Design review of the part shown in the three views and the two pictorial views. Dimensions are in mm from the part's minimum x, y and z. A direction names the side the tool comes from. Round coordinates to 2 decimals unless told otherwise and drop trailing zeros. Loops run counter-clockwise (first coordinate to the right, second up) from the corner with the lowest first, then second, coordinate; pieces in that order, holes last.
1. Tool access review of the marked faces 1 and 2: name each direction out of +Z, -Z, +X, -X, +Y, -Y from which nothing blocks a thin tool from reaching the whole face with its end or side.
2. Consider section D-D on z = 49. State the section outline as (x, y) points, then the cut area to 3 significant figures.
3. Clearance check with flat-ended pins moving along their axes: pin 1 Ø12 at (x, y) = (61, 33) entering from -Z; pin 2 Ø1 at (x, y) = (60, 45) entering from +Z; pin 3 Ø3 at (y, z) = (8.5, 97) entering from +X; pin 4 Ø10 at (x, z) = (57.5, 101.5) entering from -Y. State where each tip first meets the part, or that it passes through.
4. Consider section A-A on z = 111.5. State the section outline as (x, y) points, then the cut area to 3 significant figures.
5. To check wall thickness, follow line 1 along Z through (x, y) = (40.5, 35); line 2 along X through (y, z) = (20, 82) (1 decimal); line 3 along Z through (x, y) = (59.5, 27.5) (1 decimal). State the ranges of each line that lie inside material, in increasing order.
6. Consider section C-C on y = 5. State the section outline as (x, z) points (1 decimal).
7. Consider section B-B on x = 40. State the section outline as (y, z) points.
8. Draft analysis for pull direction Z (two halves, no side actions). For the marked faces 3, 4 and 5, state which applies: released by +Z, released by -Z, zero draft, split by the parting line, or undercut.
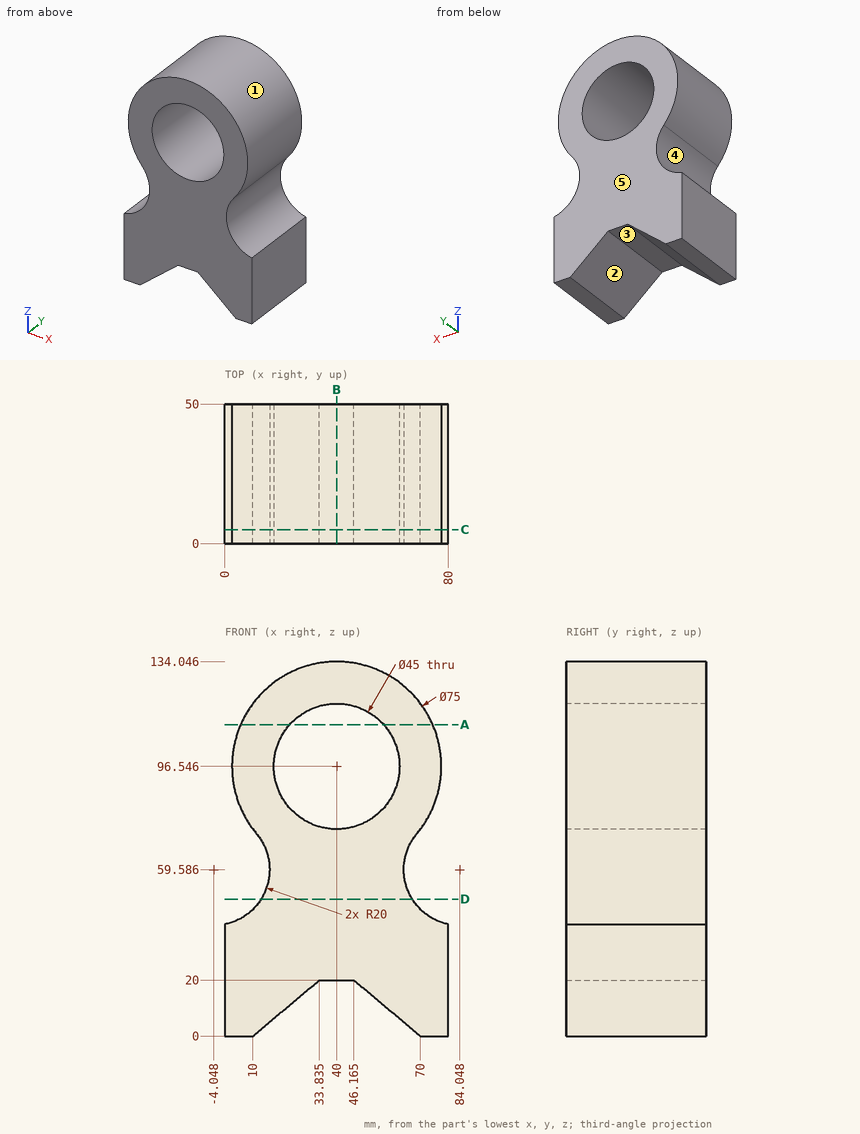
Resolved:
1. face 1: +Y, -Y
1. face 2: -Z, +Y, -Y
2. outline: (12.92, 0) - (67.08, 0) - (67.08, 50) - (12.92, 50) - close
2. area: 2,710 mm2
3. pin 1: stops at z = 2.52
3. pin 2: stops at z = 128.58
3. pin 3: stops at x = 77.5
3. pin 4: stops at y = 0
4. outline: (5.61, 0) - (23.19, 0) - (23.19, 50) - (5.61, 50) - close; (56.81, 0) - (74.39, 0) - (74.39, 50) - (56.81, 50) - close
4. area: 1,760 mm2
5. line 1: z = 20 to 74.05, 119.04 to 134.04
5. line 2: x = 5.4 to 22.8, 57.2 to 74.6
5. line 3: z = 8.8 to 85.3, 107.8 to 128.6
6. outline: (0, 0) - (10, 0) - (33.8, 20) - (46.2, 20) - (70, 0) - (80, 0) - (80, 40) arc R20 cw to (68.7, 72.4) arc R37.5 ccw (long way) to (11.3, 72.4) arc R20 cw to (0, 40) - close; hole circle Ø45 at (40, 96.5)
7. outline: (0, 20) - (50, 20) - (50, 74.05) - (0, 74.05) - close; (0, 119.05) - (50, 119.05) - (50, 134.05) - (0, 134.05) - close
8. face 3: released by -Z
8. face 4: undercut
8. face 5: zero draft
